Model file for the job. Use its own axes, mm. A direction names the side the tool comes from. Round coordinates to 2 decimals unless told otherwise and drop trailing zeros. Order: outer loops, then holes, each group sorted by start corner. A loop starts at its lowest first (then second) coordinate and runs counter-clockwise, first axis right, second up. Notation, with made-up numbers: (43.25, 9) -> (101.25, 9) arc R20 ccw to (101.25, 35) -> close; hole circle Ø7 at (-5.5, -31.75). An arc over 180 degrees is marked (long way). Answer as CSV lines item,"result".
```python
from build123d import *

# Parameters (mm, degrees)
BOSS_EXTRUDE1_DEPTH = 5.64


with BuildPart() as part:
    # Sketch1 → Boss-Extrude1 (new body)
    with BuildSketch(Plane.XY):
        with BuildLine():
            Line((652.899853243, 449.102981641), (641.00965886, 449.102981641))
            ThreePointArc((641.00965886, 449.102981641), (635.75965886, 456.212787258), (633.899853243, 464.852981641))
            Line((633.899853243, 464.852981641), (629.688308144, 464.852981641))
            Line((629.688308144, 464.852981641), (629.688308144, 460.252981641))
            Line((629.688308144, 460.252981641), (631.128193187, 460.252981641))
            Line((631.128193187, 460.252981641), (631.128193187, 457.852930641))
            Line((631.128193187, 457.852930641), (629.688308144, 457.852930641))
            Line((629.688308144, 457.852930641), (629.688308144, 455.852930641))
            Line((629.688308144, 455.852930641), (626.988308144, 455.852930641))
            Line((626.988308144, 455.852930641), (626.988308144, 457.852930641))
            Line((626.988308144, 457.852930641), (625.548423101, 457.852930641))
            Line((625.548423101, 457.852930641), (625.548423101, 460.252981641))
            Line((625.548423101, 460.252981641), (626.988308144, 460.252981641))
            Line((626.988308144, 460.252981641), (626.988308144, 464.852981641))
            Line((626.988308144, 464.852981641), (624.888308144, 464.852981641))
            Line((624.888308144, 464.852981641), (624.888308144, 470.852981641))
            Line((624.888308144, 470.852981641), (621.288308144, 470.852981641))
            Line((621.288308144, 470.852981641), (621.288308144, 464.852981641))
            Line((621.288308144, 464.852981641), (621.288308144, 424.352981641))
            Line((621.288308144, 424.352981641), (621.288308144, 418.352981641))
            Line((621.288308144, 418.352981641), (624.888308144, 418.352981641))
            Line((624.888308144, 418.352981641), (624.888308144, 424.352981641))
            Line((624.888308144, 424.352981641), (626.988308144, 424.352981641))
            Line((626.988308144, 424.352981641), (626.988308144, 428.952981641))
            Line((626.988308144, 428.952981641), (625.548423101, 428.952981641))
            Line((625.548423101, 428.952981641), (625.548423101, 431.353032641))
            Line((625.548423101, 431.353032641), (626.988308144, 431.353032641))
            Line((626.988308144, 431.353032641), (626.988308144, 433.353032641))
            Line((626.988308144, 433.353032641), (629.688308144, 433.353032641))
            Line((629.688308144, 433.353032641), (629.688308144, 431.353032641))
            Line((629.688308144, 431.353032641), (631.128193187, 431.353032641))
            Line((631.128193187, 431.353032641), (631.128193187, 428.952981641))
            Line((631.128193187, 428.952981641), (629.688308144, 428.952981641))
            Line((629.688308144, 428.952981641), (629.688308144, 424.352981641))
            Line((629.688308144, 424.352981641), (633.899853243, 424.352981641))
            ThreePointArc((633.899853243, 424.352981641), (635.75965886, 432.993176024), (641.00965886, 440.102981641))
            Line((641.00965886, 440.102981641), (652.899853243, 440.102981641))
            ThreePointArc((652.899853243, 440.102981641), (657.399853243, 444.602981641), (652.899853243, 449.102981641))
        make_face()
    extrude(amount=BOSS_EXTRUDE1_DEPTH)


solid = part.part
```
Q1. Saw through at A-A (y = 461). Write the cut outline in (x, z).
Checks:
outline,"(621.29, 0) -> (626.99, 0) -> (626.99, 5.64) -> (621.29, 5.64) -> close; (629.69, 0) -> (634.26, 0) -> (634.26, 5.64) -> (629.69, 5.64) -> close"
Q2. Saw through at D-D (y = 430). Write the cut outline in (x, z).
Checks:
outline,"(621.29, 0) -> (625.55, 0) -> (625.55, 5.64) -> (621.29, 5.64) -> close; (631.13, 0) -> (634.67, 0) -> (634.67, 5.64) -> (631.13, 5.64) -> close"
Q3. Mould opens along Y. For faces 1 (the flat face through (626, 424.353, 3)), 2 (the flat face through (625.548, 459, 3)), 3 (the flat face through (626.988, 463, 3)) say: +Y half, -Y half, draft (parallel to the pull), parting line (faces both ways), or undercut.
Checks:
face 1,"-Y half"
face 2,"undercut"
face 3,"draft"
Q4. Tool access for faces 4 (the flat face through (629.688, 463, 3)), 5 (the flat face through (624.888, 421, 3)), 6 (the flat face through (626, 428.953, 3)): list every direction of +Z, -Z, +X, -X, +Y, -Y with a clear straight run to the whole face (end or side of a thin tool).
Checks:
face 4,"+Z, -Z, +Y"
face 5,"+Z, -Z, +X, -Y"
face 6,"+Z, -Z"
Q5. Flat gauge pins, fed straight in: pin 1 (2 mm diameter, centred on x = 632.5, z = 2.5, fed in from -Y); pin 2 (0.6 mm diameter, centred on y = 432, z = 2, fed in from +X); pin 3 (1.2 mm diameter, centred on y = 430.5, z = 3, fed in from +X). Where does each tip first touch, or does it go through?
Checks:
pin 1,"y = 424.35"
pin 2,"x = 635.46"
pin 3,"x = 635.01"
Q6. Saw through at B-B (y = 466.5). Write the cut outline in (x, z), plus the area to 3 significant figures.
Checks:
outline,"(621.29, 0) -> (624.89, 0) -> (624.89, 5.64) -> (621.29, 5.64) -> close"
area,"20.3 mm²"
Q7. Wall check: L1, parallel to Y at x = 643.5, z = 2.7; L2, parallel to X at y = 468, z = 4.85; L3, parallel to X at y = 461, z = 1.5. Give the ranges that are in metal, low to high. Write a range as [from, to].
Checks:
L1,"[440.1, 449.1]"
L2,"[621.29, 624.89]"
L3,"[621.29, 626.99], [629.69, 634.26]"
Q8. Saw through at C-C (x = 651). Write the cut outline in (y, z).
Checks:
outline,"(440.1, 0) -> (449.1, 0) -> (449.1, 5.64) -> (440.1, 5.64) -> close"
